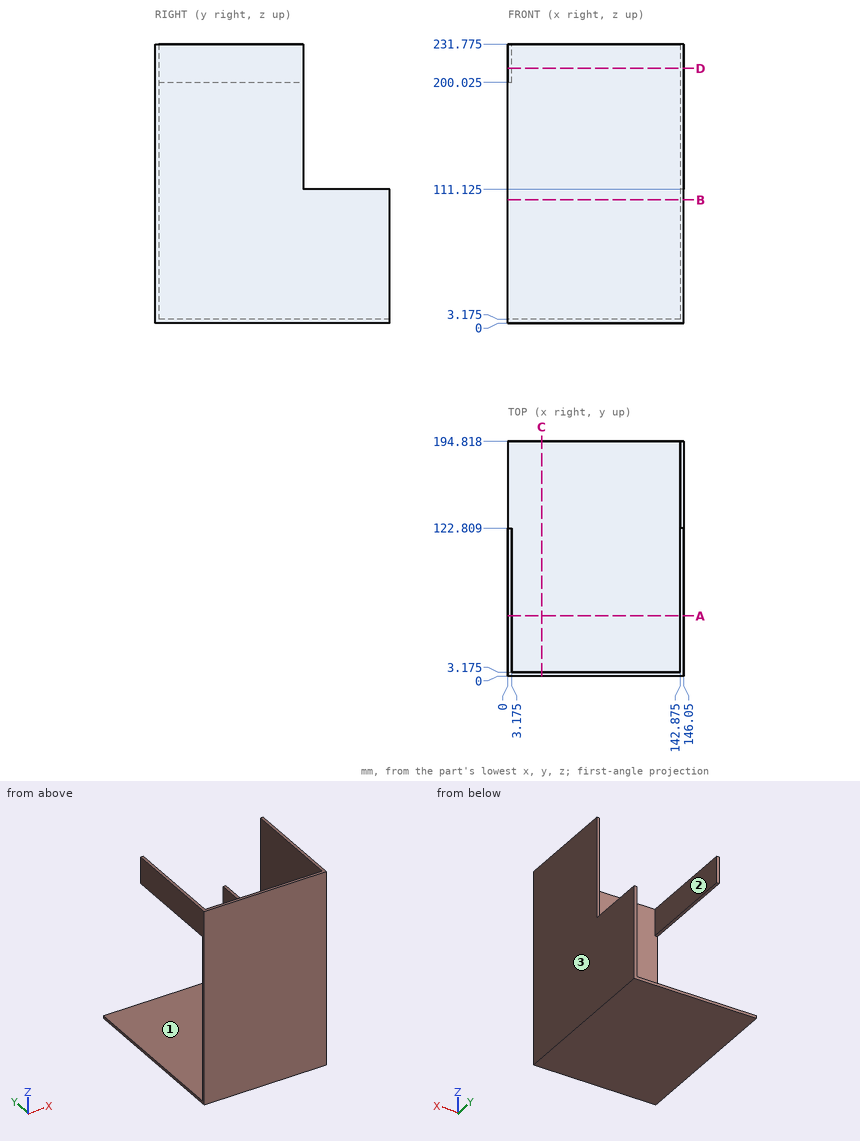
Geometry: see drawing. Coordinates: mm, zero at the bounding-box minimum. Give positions to 0.01 mm unless a question says otherwise; leave off trailing zeros. Loops run counter-clockwise (first coordinate to the right, second up) from the corner with the lowest first, then second, coordinate; pieces in that order, holes last. Notation, with made-up numbers: (9.25, -23) -> (29.25, -23) arc R12 ccw to (29.25, -9) -> close; hole circle Ø10 at (75.5, 12). An arc over 180 degrees is marked (long way). Use CSV: the item, a comma, the result in double quotes.
(1) Cut plane C-C (x = 28). Output: boundary loops of the cut face in (y, z) (3 decimals).
From the geometry:
outline,"(0, 0) -> (194.818, 0) -> (194.818, 3.175) -> (3.175, 3.175) -> (3.175, 231.775) -> (0, 231.775) -> close"
(2) First-contact query: P1, Ø5, axis at x = 93.5, z = 88, coming from the -Y side; P2, Ø1, axis at x = 144.5, z = 147.5, coming from the +Y side; P3, Ø1, axis at y = 48.5, z = 83, coming from the -X side (3 decimals); P4, Ø3, axis at x = 84.5, y = 106.5, coming from the +Z side (3 decimals). Flat tips, straight axial feed; report the tip coordinate or a pass-through.
From the geometry:
P1,"y = 0"
P2,"y = 122.81"
P3,"x = 142.875"
P4,"z = 3.175"
(3) Cut plane A-A (y = 50). Output: boundary loops of the cut face in (x, z) (3 decimals).
From the geometry:
outline,"(0, 0) -> (146.05, 0) -> (146.05, 231.775) -> (142.875, 231.775) -> (142.875, 3.175) -> (0, 3.175) -> close; (0, 200.025) -> (3.175, 200.025) -> (3.175, 231.775) -> (0, 231.775) -> close"
(4) Ray query, line 1 along X through (y, z) = (96, 48.5) (3 decimals); line 2 along Y through (x, z) = (15.5, 77.5) (3 decimals). Return the intervals inside material, ascending. Write a range as [from, to].
From the geometry:
line 1,"[142.875, 146.05]"
line 2,"[0, 3.175]"
(5) Cut plane D-D (z = 211.5). Output: boundary loops of the cut face in (x, y) (3 decimals), plus the area to 3 significant figures.
From the geometry:
outline,"(0, 0) -> (146.05, 0) -> (146.05, 122.809) -> (142.875, 122.809) -> (142.875, 3.175) -> (3.175, 3.175) -> (3.175, 122.809) -> (0, 122.809) -> close"
area,"1,220 mm^2"
(6) Pull-direction query (X, two-part tool) for the marked faces 1, 2 and 3; classes: released by +X, released by -X, zero draft, split by the parting line, or undercut.
From the geometry:
face 1,"zero draft"
face 2,"undercut"
face 3,"released by +X"
(7) Cut plane B-B (z = 102.5). Output: boundary loops of the cut face in (x, y) (3 decimals).
From the geometry:
outline,"(0, 0) -> (146.05, 0) -> (146.05, 194.818) -> (142.875, 194.818) -> (142.875, 3.175) -> (0, 3.175) -> close"
